Here's how the part is built. I have some questions about the finished solid (model axes, mm). Face numbers are marked on the shaded views. A direction names the side the tool comes from. Round coordinates to 2 decimals unless told otherwise and drop trailing zeros. Order: outer loops, then holes, each group sorted by start corner. A loop starts at its lowest first (then second) coordinate and runs counter-clockwise, first axis right, second up. Notation, with made-up numbers: (-35.75, 34.5) -> (23.25, 34.5) arc R11 ccw to (23.25, 48.5) -> close; hole circle Ø11 at (-10.75, 32). An arc over 180 degrees is marked (long way). Use a Markdown table: item, result. Add a question column.
(1) I want a section at D-D, the plane x = -5. Please give me the cut outline in (y, z).
(2) If I drill on probe 1 along Y at (x, z) = (-15.5, 0.8); probe 2 along Y at (x, z) = (-5, 0.9); probe 3 along X at (y, z) = (-1.75, 2.15), over which ranges is the centre line in solid material (lowest first)?
(3) Thinking about a two-plate mould opening in Y: for the marked faces 3, 4 and 5, which applies, pulls with the +Y half, pulls with the -Y half, needs draft (parallel to the pull), parting line crosses it, or undercut?
(4) I want a section at B-B, the plane y = 0. Please give me the cut outline in (x, z), then the cut area to 3 significant figures.
(5) I want a section at A-A, the plane x = -10. Please give me the cut outline in (y, z).
(6) I'm going to push a flat-ended pin straight in: P1, Ø4.5, axis at x = -5, y = 0, coming from the -Z side. Where does the tip first touch, or does it pass through?
(7) I want a section at C-C, the plane z = 2.75. Please give me the cut outline in (x, y), then the cut area to 3 significant figures.
(8) On a 3-axis mill with a long thin cutter (end or side, diameter ignored), from which of +Z, -Z, +X, -X, +Y, -Y can I reach the whole of each face in a straight line? I mean the marked faces 1 and 2. Say none if no direction works.
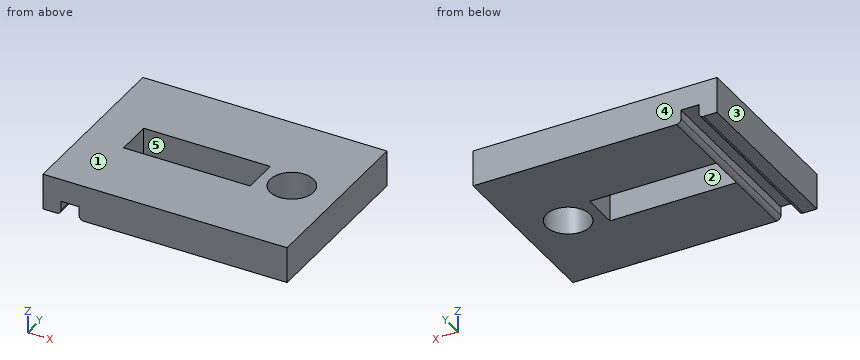
from build123d import *

# Parameters (mm, degrees)
F1_DEPTH      = 9.9
F1_DEPTH_BACK = 9.9
F2_R          = 2.4
F3_DEPTH      = 4.001
F4_R          = 0.5
F5_W          = 14
F5_H          = 4
F6_DEPTH      = 4.001


with BuildPart() as f1:
    # F0 (on Front) → F1 (new body, two sides)
    with BuildSketch(Plane.XZ) as f1_sk:
        Polygon((-23, 0), (0, 0), (0, 4), (-27, 4), (-27, 0), (-25, 0), (-25, 1.5), (-23, 1.5), align=None)
    extrude(amount=F1_DEPTH)
    extrude(f1_sk.sketch, amount=-F1_DEPTH_BACK)

    # F2 (on face) → F3 (cut, through all)
    with BuildSketch(Plane.XY.offset(4)):
        with Locations((-5, 0)):
            Circle(F2_R)
    extrude(amount=-F3_DEPTH, mode=Mode.SUBTRACT)

    # F4
    f4_edges = [f1.edges().sort_by_distance(p)[0] for p in [
        (-25, 0, 0),
        (-23, 0, 0),
    ]]
    fillet(f4_edges, radius=F4_R)

    # F5 (on face) → F6 (cut, through all)
    with BuildSketch(Plane(origin=(0, 0, 0), x_dir=(1, 0, 0), z_dir=(0, 0, -1))):
        with Locations((-15.5, 0)):
            Rectangle(F5_W, F5_H)
    extrude(amount=-F6_DEPTH, mode=Mode.SUBTRACT)


solid = f1.part
Taken from the geometry:
| question | item | result |
|---|---|---|
| 1 | outline | (-9.9, 0) -> (-2.4, 0) -> (-2.4, 4) -> (-9.9, 4) -> close; (2.4, 0) -> (9.9, 0) -> (9.9, 4) -> (2.4, 4) -> close |
| 2 | probe 1 | y = -9.9 to -2, 2 to 9.9 |
| 2 | probe 2 | y = -9.9 to -2.4, 2.4 to 9.9 |
| 2 | probe 3 | x = -27 to -22.5, -8.5 to -6.64, -3.36 to 0 |
| 3 | face 3 | needs draft |
| 3 | face 4 | pulls with the +Y half |
| 3 | face 5 | undercut |
| 4 | outline | (-27, 0) -> (-25.5, 0) arc R0.5 ccw to (-25, 0.5) -> (-25, 1.5) -> (-23, 1.5) -> (-23, 0.5) arc R0.5 ccw to (-22.5, 0) -> (-22.5, 4) -> (-27, 4) -> close; (-8.5, 0) -> (-7.4, 0) -> (-7.4, 4) -> (-8.5, 4) -> close; (-2.6, 0) -> (0, 0) -> (0, 4) -> (-2.6, 4) -> close |
| 4 | area | 29.7 mm2 |
| 5 | outline | (-9.9, 0) -> (-2, 0) -> (-2, 4) -> (-9.9, 4) -> close; (2, 0) -> (9.9, 0) -> (9.9, 4) -> (2, 4) -> close |
| 6 | P1 | passes through |
| 7 | outline | (-27, -9.9) -> (0, -9.9) -> (0, 9.9) -> (-27, 9.9) -> close; hole (-22.5, -2) -> (-8.5, -2) -> (-8.5, 2) -> (-22.5, 2) -> close; hole circle Ø4.8 at (-5, 0) |
| 7 | area | 461 mm2 |
| 8 | face 1 | +Z, +X, -X, +Y, -Y |
| 8 | face 2 | +Z, -Z |
